from build123d import *

# Parameters (mm, degrees)
F0_W     = 560.33
F0_H     = 532.76
F0_W_2   = 5.08
F0_H_2   = 161.7
F0_W_3   = 15.6
F0_H_3   = 333.4
F0_W_4   = 6.03
F0_H_4   = 244.5
F0_W_5   = 120
F0_H_5   = 165.1
F0_W_6   = 76.2
F0_W_7   = 168.3
F0_H_6   = 512.76
F0_W_8   = 6.35
F0_W_9   = 30.5
F0_H_7   = 512.8
F0_W_10  = 40.89
F0_H_8   = 66.7
F0_H_9   = 93.309008
F0_W_11  = 38.09
F0_W_12  = 206.2
F0_H_10  = 163.5
F0_H_11  = 83.89079
F0_H_12  = 164.569237
F1_DEPTH = 650
F2_W     = 10
F2_H     = 532.76
F3_DEPTH = 560.33
F4_W     = 560.33
F4_H     = 9.96
F4_H_2   = 10
F5_DEPTH = 10


with BuildPart() as f1:
    # F0 (on Front) → F1 (new body)
    with BuildSketch(Plane.XZ):
        with Locations((-1.447709, 27.52879)):
            Rectangle(F0_W, F0_H)
        with Locations((-74.422709, -148.00121)):
            Rectangle(F0_W_2, F0_H_2, mode=Mode.SUBTRACT)
        with Locations((-43.872709, -62.15121)):
            Rectangle(F0_W_3, F0_H_3, mode=Mode.SUBTRACT)
        with Locations((-74.422709, 23.69879)):
            Rectangle(F0_W_2, F0_H_2, mode=Mode.SUBTRACT)
        with Locations((17.442291, -106.60121)):
            Rectangle(F0_W_4, F0_H_4, mode=Mode.SUBTRACT)
        with Locations((33.472291, -106.60121)):
            Rectangle(F0_W_4, F0_H_4, mode=Mode.SUBTRACT)
        with Locations((49.502291, -106.60121)):
            Rectangle(F0_W_4, F0_H_4, mode=Mode.SUBTRACT)
        with Locations((122.517291, -146.30121)):
            Rectangle(F0_W_5, F0_H_5, mode=Mode.SUBTRACT)
        with Locations((230.617291, -146.30121)):
            Rectangle(F0_W_6, F0_H_5, mode=Mode.SUBTRACT)
        with Locations((-187.462709, 27.52879)):
            Rectangle(F0_W_7, F0_H_6, mode=Mode.SUBTRACT)
        with Locations((-90.137709, 27.52879)):
            Rectangle(F0_W_8, F0_H_6, mode=Mode.SUBTRACT)
        with Locations((-10.822709, 27.54879)):
            Rectangle(F0_W_9, F0_H_7, mode=Mode.SUBTRACT)
        with Locations((-56.517709, 147.249782)):
            Rectangle(F0_W_10, F0_H_8, mode=Mode.SUBTRACT)
        with Locations((-56.517709, 237.254286)):
            Rectangle(F0_W_10, F0_H_9, mode=Mode.SUBTRACT)
        with Locations((33.472291, 107.508)):
            Rectangle(F0_W_11, F0_H_5, mode=Mode.SUBTRACT)
        with Locations((165.617291, 27.629553)):
            Rectangle(F0_W_12, F0_H_10, mode=Mode.SUBTRACT)
        with Locations((33.472291, 242.003395)):
            Rectangle(F0_W_11, F0_H_11, mode=Mode.SUBTRACT)
        with Locations((165.617291, 201.664171)):
            Rectangle(F0_W_12, F0_H_12, mode=Mode.SUBTRACT)
    extrude(amount=F1_DEPTH)

    # F2 (on face) → F3 (join, through all)
    with BuildSketch(Plane(origin=(-281.612709, 0, 0), x_dir=(0, -1, 0), z_dir=(-1, 0, 0))):
        with Locations((-5, 27.52879)):
            Rectangle(F2_W, F2_H)
    extrude(amount=-F3_DEPTH)

    # F4 (on face) → F5 (join)
    with BuildSketch(Plane.XZ.offset(650)):
        with Locations((-1.447709, 288.92879)):
            Rectangle(F4_W, F4_H)
        with Locations((-1.447709, -233.85121)):
            Rectangle(F4_W, F4_H_2)
    extrude(amount=F5_DEPTH)


solid = f1.part
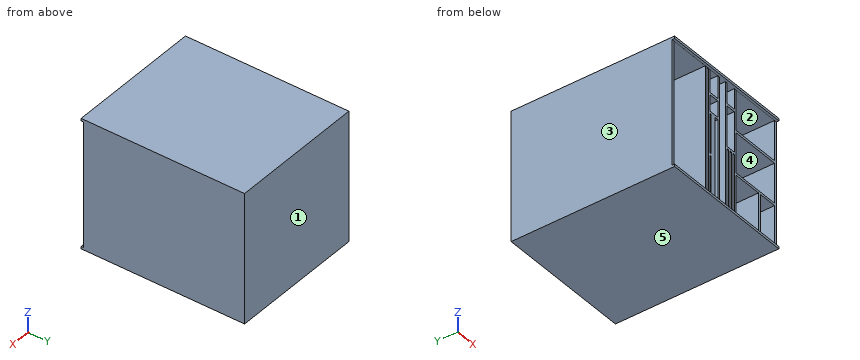
Source: CAD feature listing. Evaluate the final solid. Frame: model axes, mm. Face numbers are marked on the shaded views. A direction names the side the tool comes from. Coordinates: 2 decimals unless noted, no trailing zeros. Order: outer loops, then holes, each group sorted by start corner. A loop starts at its lowest first (then second) coordinate and runs counter-clockwise, first axis right, second up.
Item 1: Cut plane C-C (y = -601). Count the separate pieces of the cut face and the enclosed holes in it, plus the area to 3 significant figures.
Output values:
separate pieces: 1
enclosed holes: 17
area: 66,000 mm2
Item 2: Material intervals for line 1 (Z direction, x = 98, y = -77); line 2 (X direction, y = -459, z = 105); line 3 (X direction, y = -557, z = 119), sorted ascending.
Output values:
line 1: z = -238.85 to -228.85, -63.75 to -54.12, 109.38 to 119.38, 283.95 to 293.91
line 2: x = -281.61 to -271.61, -103.31 to -93.31, -86.96 to -26.07, 4.43 to 14.43, 52.52 to 62.52, 268.72 to 278.72
line 3: x = -281.61 to -271.61, -103.31 to -93.31, -86.96 to -76.96, -36.07 to -26.07, 4.43 to 14.43, 52.52 to 278.72
Item 3: Cut plane A-A (z = 238). Return loops of the section in (x, y).
Output values:
outline: (-281.61, -650) - (-271.61, -650) - (-271.61, 0) - (-103.31, 0) - (-103.31, -650) - (-93.31, -650) - (-93.31, 0) - (-86.96, 0) - (-86.96, -650) - (-76.96, -650) - (-76.96, 0) - (-36.07, 0) - (-36.07, -650) - (-26.07, -650) - (-26.07, 0) - (4.43, 0) - (4.43, -650) - (14.43, -650) - (14.43, 0) - (52.52, 0) - (52.52, -650) - (62.52, -650) - (62.52, 0) - (268.72, 0) - (268.72, -650) - (278.72, -650) - (278.72, 10) - (-281.61, 10) - close
Item 4: Set-up query: the marked faces 1 and 2. Return all of +Z, -Z, +X, -X, +Y, -Y with unobstructed straight access to the full face (end or side cutting, diameter ignored); none if empty.
Output values:
face 1: +Z, -Z, +X, -X, +Y
face 2: -Y
Item 5: Pull-direction query (X, two-part tool) for the marked faces 3, 4 and 5; classes: pulls with the +X half, pulls with the -X half, needs draft (parallel to the pull), parting line crosses it, or undercut.
Output values:
face 3: pulls with the -X half
face 4: undercut
face 5: needs draft
Item 6: First-contact query: P1, Ø12, axis at x = 120.5, z = 111.5, coming from the -Y side; P2, Ø5, axis at x = 48.5, z = 185, coming from the -Y side. Flat tips, straight axial feed; report the tip coordinate or a pass-through.
Output values:
P1: stops at y = -650
P2: stops at y = 0
Item 7: Cut plane B-B (x = 162.5). Return loops of the section in (y, z).
Output values:
outline: (-660, -238.85) - (10, -238.85) - (10, 293.91) - (-660, 293.91) - (-660, 283.95) - (0, 283.95) - (0, 119.38) - (-650, 119.38) - (-650, 109.38) - (0, 109.38) - (0, -54.12) - (-650, -54.12) - (-650, -63.75) - (0, -63.75) - (0, -228.85) - (-660, -228.85) - close
